```python
from build123d import *

# Parameters (mm, degrees)
SKETCH1_W               = 38
SKETCH1_H               = 22
PCB_DEPTH               = 1.6
MOUNT_HOLE_1_DEPTH      = 44.938138331
MOUNT_HOLE_1_DEPTH_BACK = 44.938138331
SKETCH2_R               = 1.5
MOUNT_HOLE_2_DEPTH      = 44.938138331
MOUNT_HOLE_2_DEPTH_BACK = 44.938138331
SKETCH3_R               = 1.5
DS3231_IC_START         = 1.6
SKETCH4_W               = 10.3
SKETCH4_H               = 7.5
DS3231_IC_DEPTH         = 2.5
AT24C32_EEPROM_START    = 1.6
SKETCH5_W               = 5
SKETCH5_H               = 4
AT24C32_EEPROM_DEPTH    = 1.5
HEADER_6PIN_START       = 1.6
SKETCH6_W               = 2.5
SKETCH6_H               = 15.2
HEADER_6PIN_DEPTH       = 8.5
SKETCH7_R               = 11
CR2032_HOLDER_DEPTH     = 5.5


with BuildPart() as part:
    # Sketch1 → PCB (new body)
    with BuildSketch(Plane(origin=(0, 0, 0), x_dir=(1, 0, 0), z_dir=(0, 1, 0))):
        with Locations((19, 11)):
            Rectangle(SKETCH1_W, SKETCH1_H)
    extrude(amount=PCB_DEPTH)

    # Sketch2 → Mount_hole_1 (cut, two sides: drawn at the far end of the back side and taken through both)
    with BuildSketch(Plane(origin=(0, 0, 0), x_dir=(1, 0, 0), z_dir=(0, 1, 0)).offset(-MOUNT_HOLE_1_DEPTH_BACK)):
        with Locations(Location((2.5, 19.5, 0), (0, 0, 270))):
            Circle(SKETCH2_R)
    extrude(amount=MOUNT_HOLE_1_DEPTH + MOUNT_HOLE_1_DEPTH_BACK, mode=Mode.SUBTRACT)

    # Sketch3 → Mount_hole_2 (cut, two sides: drawn at the far end of the back side and taken through both)
    with BuildSketch(Plane(origin=(0, 0, 0), x_dir=(1, 0, 0), z_dir=(0, 1, 0)).offset(-MOUNT_HOLE_2_DEPTH_BACK)):
        with Locations(Location((2.5, 2.5, 0), (0, 0, 270))):
            Circle(SKETCH3_R)
    extrude(amount=MOUNT_HOLE_2_DEPTH + MOUNT_HOLE_2_DEPTH_BACK, mode=Mode.SUBTRACT)

    # Sketch4 → DS3231_IC (add)
    with BuildSketch(Plane(origin=(0, 0, 0), x_dir=(1, 0, 0), z_dir=(0, 1, 0)).offset(DS3231_IC_START)):
        with Locations((14.15, 8.75)):
            Rectangle(SKETCH4_W, SKETCH4_H)
    extrude(amount=DS3231_IC_DEPTH)

    # Sketch5 → AT24C32_EEPROM (add)
    with BuildSketch(Plane(origin=(0, 0, 0), x_dir=(1, 0, 0), z_dir=(0, 1, 0)).offset(AT24C32_EEPROM_START)):
        with Locations((24.5, 9)):
            Rectangle(SKETCH5_W, SKETCH5_H)
    extrude(amount=AT24C32_EEPROM_DEPTH)

    # Sketch6 → Header_6pin (add)
    with BuildSketch(Plane(origin=(0, 0, 0), x_dir=(1, 0, 0), z_dir=(0, 1, 0)).offset(HEADER_6PIN_START)):
        with Locations((36.25, 11)):
            Rectangle(SKETCH6_W, SKETCH6_H)
    extrude(amount=HEADER_6PIN_DEPTH)

    # Sketch7 → CR2032_holder (add)
    with BuildSketch(Plane(origin=(0, 0, 0), x_dir=(1, 0, 0), z_dir=(0, 1, 0))):
        with Locations(Location((19, 11, 0), (0, 0, 270))):
            Circle(SKETCH7_R)
    extrude(amount=-CR2032_HOLDER_DEPTH)


solid = part.part
```
Can you work these out from the model? Positions are in its coordinate system, mm. A direction names the side the tool comes from. Round coordinates to 2 decimals unless told otherwise and drop trailing zeros. Loops run counter-clockwise (first coordinate to the right, second up) from the corner with the lowest first, then second, coordinate; pieces in that order, holes last.
Item 1: Suppose I cut it at B-B, the plane y = 2.5. Write out the boundary of the cut face in (x, z).
Item 2: Which directions (+Z, -Z, +X, -X, +Y, -Y) give clear straight access to the entire face, cutting with the end or side of a thin tool? Please do faces 5 (the flat face through (37.5, 6, -11)), 6 (the cylindrical face through (8.26, -2.71, -13.38)), 7 (the flat face through (14, 3, -12.5)).
Item 3: Suppose I cut it at C-C, the plane z = -19.5. Write out the boundary of the cut face in (x, y), then the cut area to 3 significant figures.
Item 4: If we mould it in two halves opening along Z, with no side actions, what happens to faces 1 (the flat face through (24, 2, -11)), 2 (the flat face through (9, 3, -9)), 3 (the flat face through (36, 6, -3.4)), 4 (the cylindrical face through (1.17, 0.79, -1.81))? For each: +Z half, -Z half, draft (parallel to the pull), parting line (faces both ways), or undercut.
Item 5: Please list where these lines run through material, in increasing order: L1, parallel to Z at x = 2.5, y = 1; L2, parallel to X at y = 1, z = -19.5; L3, parallel to X at y = 3.5, z = -6.75.
Item 6: Suppose I cut it at A-A, the plane x = 2.5. Write out the boundary of the cut face in (y, z), then the cut area to 3 significant figures.
Item 7: Suppose I cut it at D-D, the plane z = -6.5. Write out the boundary of the cut face in (x, y), then the cut area to 3 significant figures.
Item 8: Will these pins go through, and if not, where does the flat tip stop? pin 1 Ø5 at (x, z) = (6, -3) entering from -Y; pin 2 Ø1.2 at (y, z) = (2.5, -9.5) entering from -X; pin 3 Ø5.5 at (x, z) = (32.5, -9) entering from -Y; pin 4 Ø1.5 at (x, z) = (22.5, -9.5) entering from +Y.
Reported:
1. outline: (9, -12.5) - (19.3, -12.5) - (19.3, -5) - (9, -5) - close; (22, -11) - (27, -11) - (27, -7) - (22, -7) - close; (35, -18.6) - (37.5, -18.6) - (37.5, -3.4) - (35, -3.4) - close
2. face 5: +Z, -Z, +X, +Y
2. face 6: -Y
2. face 7: -Z, -X, +Y
3. outline: (0, 0) - (1, 0) - (1, 1.6) - (0, 1.6) - close; (4, 0) - (12.02, 0) - (12.02, -5.5) - (25.98, -5.5) - (25.98, 0) - (38, 0) - (38, 1.6) - (4, 1.6) - close
3. area: 133 mm2
4. face 1: -Z half
4. face 2: draft
4. face 3: +Z half
4. face 4: undercut
5. L1: z = -22 to -21, -18 to -4, -1 to 0
5. L2: x = 0 to 1, 4 to 38
5. L3: x = 9 to 19.3, 35 to 37.5
6. outline: (0, -22) - (1.6, -22) - (1.6, -21) - (0, -21) - close; (0, -18) - (1.6, -18) - (1.6, -4) - (0, -4) - close; (0, -1) - (1.6, -1) - (1.6, 0) - (0, 0) - close
6. area: 25.6 mm2
7. outline: (0, 0) - (8.96, 0) - (8.96, -5.5) - (29.04, -5.5) - (29.04, 0) - (38, 0) - (38, 1.6) - (37.5, 1.6) - (37.5, 10.1) - (35, 10.1) - (35, 1.6) - (19.3, 1.6) - (19.3, 4.1) - (9, 4.1) - (9, 1.6) - (0, 1.6) - close
7. area: 218 mm2
8. pin 1: stops at y = 0
8. pin 2: stops at x = 9
8. pin 3: stops at y = -5.5
8. pin 4: stops at y = 3.1
